Build history of the part. All positions in model axes, mm. Round coordinates to 2 decimals unless told otherwise and drop trailing zeros. Write each loop counter-clockwise with the first axis right and the second up, starting at its lowest first coordinate (ties: lowest second). Pieces come first, ordered by that corner, then holes.
1) Saw through at A-A (z = 3). Write the cut outline in (x, y).
2) Wall check: probe 1 along Y at (x, z) = (-0.5, 3); probe 2 along Y at (x, z) = (13, 2); probe 3 along Z at (x, y) = (-8, 0). Give the ranges that are in metal, low to high.
3) Flat gauge pin, fed straight in: pin 1 (2 mm diameter, centred on y = 0, z = 3, fed in from +X). Where does the tip first touch, or does it go through?
4) Saw through at B-B (x = -14). Write the cut outline in (y, z).
Autodesk Inventor part; units mm, degrees
ref_plane "YZ Plane" through (0, 0, 0) normal (1, 0, 0) x (0, 1, 0)
ref_plane "XZ Plane" through (0, 0, 0) normal (0, 1, 0) x (-1, 0, 0)
ref_plane "XY Plane" through (0, 0, 0) normal (0, 0, 1) x (1, 0, 0)
sketch "スケッチ1" plane through (0, 0, 0) normal (0, 0, 1) x (1, 0, 0)
  line L0 (25.5, 80) -> (-25.5, 80)
  line L1 (-25.5, 80) -> (-25.5, 60.7746)
  line L2 (-25.5, -80) -> (25.5, -80)
  line L3 (25.5, -80) -> (25.5, -60.7746)
  line L4 (25.5, 80) -> (-25.5, -80) construction
  line L5 (-25.5, 80) -> (25.5, -80) construction
  arc A0 (-25.5, 0.7746) -> (-25.5, -0.7746) centre (-26.9, 0) ccw construction
  arc A1 (-25.5, 60.7746) -> (-25.5, 59.2254) centre (-26.9, 60) ccw construction
  arc A2 (-25.5, -59.2254) -> (-25.5, -60.7746) centre (-26.9, -60) ccw construction
  arc A3 (25.5, 0.7746) -> (25.5, -0.7746) centre (26.9, 0) ccw
  arc A4 (25.5, 60.7746) -> (25.5, 59.2254) centre (26.9, 60) ccw
  arc A5 (25.5, -60.7746) -> (25.5, -59.2254) centre (26.9, -60) ccw construction
  arc A6 (-25.5, 59.2254) -> (-25.5, 60.7746) centre (-26.9, 60) ccw
  line L6 (-25.5, 60.7746) -> (-25.5, 59.2254) construction
  line L7 (-25.5, 59.2254) -> (-25.5, 0.7746)
  arc A7 (-25.5, -0.7746) -> (-25.5, 0.7746) centre (-26.9, 0) ccw
  line L8 (-25.5, -0.7746) -> (-25.5, -59.2254)
  line L9 (-25.5, 0.7746) -> (-25.5, -0.7746) construction
  line L10 (-25.5, -59.2254) -> (-25.5, -60.7746) construction
  line L11 (-25.5, -60.7746) -> (-25.5, -80)
  arc A8 (-25.5, -60.7746) -> (-25.5, -59.2254) centre (-26.9, -60) ccw
  arc A9 (25.5, -59.2254) -> (25.5, -60.7746) centre (26.9, -60) ccw
  line L12 (25.5, -60.7746) -> (25.5, -59.2254) construction
  line L13 (25.5, -59.2254) -> (25.5, -0.7746)
  arc A10 (25.5, -0.7746) -> (25.5, 0.7746) centre (26.9, 0) ccw construction
  line L14 (25.5, -0.7746) -> (25.5, 0.7746) construction
  line L15 (25.5, 0.7746) -> (25.5, 59.2254)
  arc A11 (25.5, 59.2254) -> (25.5, 60.7746) centre (26.9, 60) ccw construction
  line L16 (25.5, 59.2254) -> (25.5, 60.7746) construction
  line L17 (25.5, 60.7746) -> (25.5, 80)
  point P0 (0, 0)
  point P1 (0, 0)
  point P2 (0, 0)
  dimension "d0" = 51
  dimension "d1" = 160
  dimension "d2" = 3.2
  dimension "d3" = 3.2
  dimension "d4" = 3.2
  dimension "d5" = 60
  dimension "d6" = 60
  dimension "d7" = 3.2
  dimension "d8" = 3.2
  dimension "d9" = 3.2
  dimension "d10" = 60
  dimension "d11" = 60
  dimension "d12" = 1.4
  dimension "d13" = 1.4
extrude "押し出し1" add sketch "スケッチ1" along normal blind 6
sketch "スケッチ2" plane through (25.5, 0.7746, 0) normal (1, 0, 0) x (0, 0, -1)
  circle A0 centre (-3, -0.7746) radius 1.25
  circle A1 centre (-3, 59.2254) radius 1.25
  circle A2 centre (-3, -60.7746) radius 1.25
  point P0 (0, -0.7746)
  dimension "d16" = 2.5
  dimension "d17" = 2.5
  dimension "d18" = 2.5
  dimension "d19" = 60
  dimension "d20" = 60
  dimension "d21" = 3
extrude "押し出し2" cut sketch "スケッチ2" against normal through all
fillet "フィレット1" radius 2 4 edges at (25.5, 80, 3) (-25.5, 80, 3) (25.5, -80, 3) (-25.5, -80, 3)
properties part number "関節3_上板" material "ポリカーボネート、スモーク"
Evaluation:
1. outline: (-25.5, -78) arc R2 ccw to (-23.5, -80) - (23.5, -80) arc R2 ccw to (25.5, -78) - (25.5, -61.25) - (-25.5, -61.25) - close; (-25.5, -58.75) - (25.5, -58.75) - (25.5, -1.25) - (-25.5, -1.25) - close; (-25.5, 1.25) - (25.5, 1.25) - (25.5, 58.75) - (-25.5, 58.75) - close; (-25.5, 61.25) - (25.5, 61.25) - (25.5, 78) arc R2 ccw to (23.5, 80) - (-23.5, 80) arc R2 ccw to (-25.5, 78) - close
2. probe 1: y = -80 to -61.25, -58.75 to -1.25, 1.25 to 58.75, 61.25 to 80
2. probe 2: y = -80 to -60.75, -59.25 to -0.75, 0.75 to 59.25, 60.75 to 80
2. probe 3: z = 0 to 1.75, 4.25 to 6
3. pin 1: passes through
4. outline: (-80, 0) - (80, 0) - (80, 6) - (-80, 6) - close; hole circle Ø2.5 at (-60, 3); hole circle Ø2.5 at (0, 3); hole circle Ø2.5 at (60, 3)
